Here's how the part is built. I have some questions about the finished solid (model axes, mm). Coordinates: 2 decimals unless noted, no trailing zeros. Write each loop counter-clockwise with the first axis right and the second up, starting at its lowest first coordinate (ties: lowest second). Pieces come first, ordered by that corner, then holes.
from build123d import *

# Parameters (mm, degrees)
ESQUISSE1_R        = 9.6
ESQUISSE1_R_2      = 7
BOSS_EXTRU_1_DEPTH = 9
CHANFREIN5_SIZE    = 0.9
CHANFREIN5_SIZE2   = 1.558845727
CHANFREIN9_SIZE    = 0.9
CHANFREIN9_SIZE2   = 1.558845727


with BuildPart() as part:
    # Esquisse1 → Boss.-Extru.1 (new body)
    with BuildSketch(Plane.XY):
        Circle(ESQUISSE1_R)
        Circle(ESQUISSE1_R_2, mode=Mode.SUBTRACT)
    extrude(amount=BOSS_EXTRU_1_DEPTH)

    # Chanfrein5
    chanfrein5_edges = [part.edges().sort_by_distance(p)[0] for p in [
        (-9.6, 0, 9),
    ]]
    chanfrein5_side = [part.faces().sort_by_distance(p)[0] for p in [
        (-9.6, 0, 4.5),
    ]]
    chamfer(chanfrein5_edges, length=CHANFREIN5_SIZE, length2=CHANFREIN5_SIZE2, reference=chanfrein5_side[0])

    # Chanfrein9
    chanfrein9_edges = [part.edges().sort_by_distance(p)[0] for p in [
        (-9.6, 0, 0),
    ]]
    chanfrein9_side = [part.faces().sort_by_distance(p)[0] for p in [
        (-9.6, 0, 4.05),
    ]]
    chamfer(chanfrein9_edges, length=CHANFREIN9_SIZE, length2=CHANFREIN9_SIZE2, reference=chanfrein9_side[0])


solid = part.part
1. I want a section at A-A (y = 0). List the corners of the cut face in (x, z) for me, then the cut area to 3 significant figures.
2. Thinking about a two-plate mould opening in Y: for faces 1 (the face through (5.161, 8.095, 4.45)), 2 (the face through (-2, 7, 9)), 3 (the face through (6.466, -2.681, 4.437)), which applies, pulls with the +Y half, pulls with the -Y half, needs draft (parallel to the pull), parting line crosses it, or undercut?
3. If I drill on line 1 (Y direction, x = 0, z = 2); line 2 (X direction, y = 6, z = 7.75); line 3 (X direction, y = 3.5, z = 8.75), over which ranges is the centre line in solid material (lowest first)?
4. I want a section at C-C (z = 3.75). List the corners of the cut face in (x, y) for me.
5. For pin 1 Ø1.5 at (y, z) = (1, 5.5) entering from +X; pin 2 Ø1 at (y, z) = (-7, 4.5) entering from -X; pin 3 Ø2 at (x, z) = (3, 1) entering from -Y, each with a flat end and sliding along its axis, tell me the tip position at first contact or that it passes through.
Response values:
1. outline: (-9.6, 0.9) - (-8.04, 0) - (-7, 0) - (-7, 9) - (-8.04, 9) - (-9.6, 8.1) - close; (7, 0) - (8.04, 0) - (9.6, 0.9) - (9.6, 8.1) - (8.04, 9) - (7, 9) - close
1. area: 44.0 mm2
2. face 1: parting line crosses it
2. face 2: needs draft
2. face 3: undercut
3. line 1: y = -9.6 to -7, 7 to 9.6
3. line 2: x = -7.49 to -3.61, 3.61 to 7.49
3. line 3: x = -7.72 to -6.06, 6.06 to 7.72
4. outline: circle Ø19.2 at (0, 0); hole circle Ø14 at (0, 0)
5. pin 1: stops at x = 9.6
5. pin 2: stops at x = -7.06
5. pin 3: stops at y = -9.39
